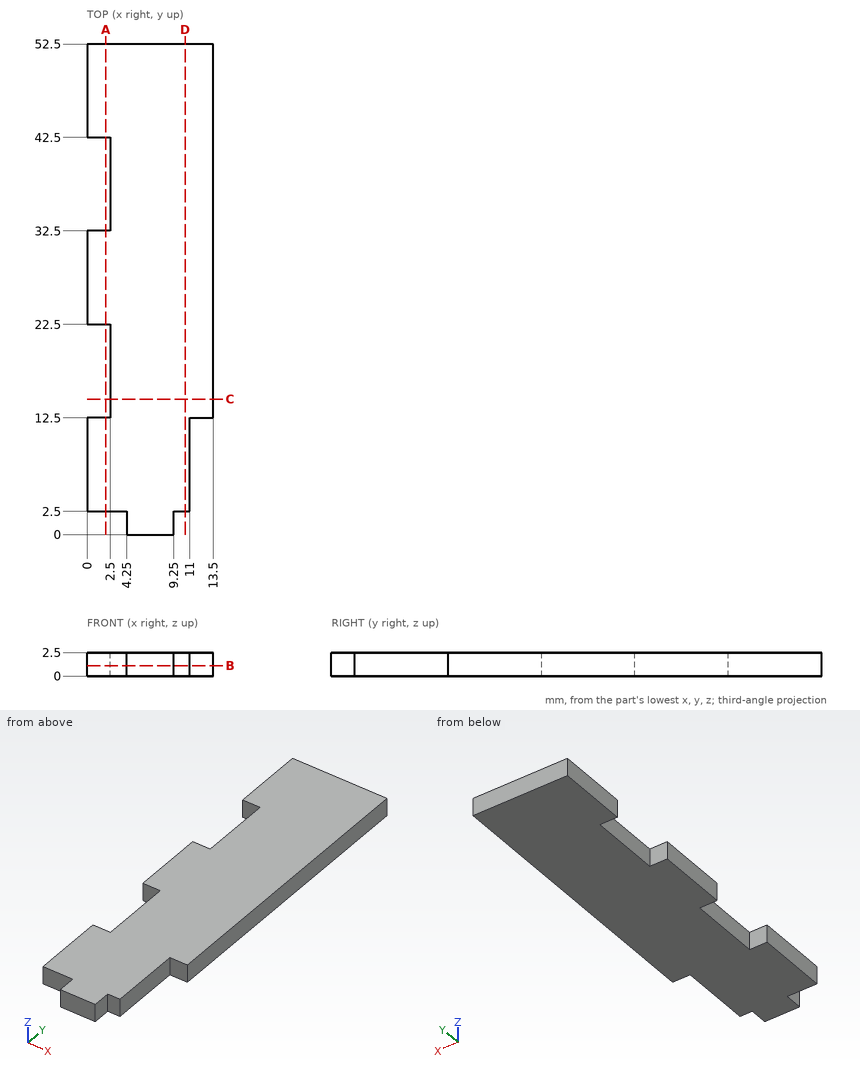
Design review of the part shown in the three views and the two pictorial views. Dimensions are in mm from the part's minimum x, y and z. Give positions to 0.01 mm unless a question says otherwise; leave off trailing zeros. Write each loop counter-clockwise with the first axis right and the second up, starting at its lowest first coordinate (ties: lowest second). Pieces come first, ordered by that corner, then holes. Notation, with made-up numbers: M 79.25,75 L 97.25,75 A26 cw 97.25,102 Z; hole C 26,23.5 d9. An arc over 180 degrees is marked long. One line per item, written item: value.
1) Take a section at D-D, the plane x = 10.5. Write out the cut boundary in (y, z).
Results are:
outline: M 2.5,0 L 52.5,0 L 52.5,2.5 L 2.5,2.5 Z
2) Take a section at A-A, the plane x = 2. Write out the cut boundary in (y, z).
Results are:
outline: M 2.5,0 L 12.5,0 L 12.5,2.5 L 2.5,2.5 Z; M 22.5,0 L 32.5,0 L 32.5,2.5 L 22.5,2.5 Z; M 42.5,0 L 52.5,0 L 52.5,2.5 L 42.5,2.5 Z
3) For P1, Ø1.2, axis at y = 7, z = 1.5, coming from the +X side; P2, Ø1.2, axis at x = 2, z = 0.5, coming from the -Y side; P3, Ø1.2, axis at y = 19, z = 1, coming from the -X side, all flat-tipped, find the tip position at first contact; note any pin that passes through.
Results are:
P1: stops at x = 11
P2: stops at y = 2.5
P3: stops at x = 2.5
4) Take a section at B-B, the plane z = 1.1. Write out the cut boundary in (x, y).
Results are:
outline: M 0,2.5 L 4.25,2.5 L 4.25,0 L 9.25,0 L 9.25,2.5 L 11,2.5 L 11,12.5 L 13.5,12.5 L 13.5,52.5 L 0,52.5 L 0,42.5 L 2.5,42.5 L 2.5,32.5 L 0,32.5 L 0,22.5 L 2.5,22.5 L 2.5,12.5 L 0,12.5 Z
5) Take a section at C-C, the plane y = 14.5. Write out the cut boundary in (x, z).
Results are:
outline: M 2.5,0 L 13.5,0 L 13.5,2.5 L 2.5,2.5 Z
6) For line 1 (Y direction, x = 0.75, z = 0.9); line 2 (X direction, y = 6.5, z = 0.65); line 3 (X direction, y = 38.5, z = 0.95), list the stretches that pass through material, from the lowest coordinate up. Write a range as from..to.
Results are:
line 1: y = 2.5..12.5, 22.5..32.5, 42.5..52.5
line 2: x = 0..11
line 3: x = 2.5..13.5
